Job drawing, mm, ordinate dimensions from the low corner. One solid piece. Give positions to 0.01 mm unless a question says otherwise; leave off trailing zeros. Order: outer loops, then holes, each group sorted by start corner. A loop starts at its lowest first (then second) coordinate and runs counter-clockwise, first axis right, second up. Notation, with made-up numbers: (76, 4.5) -> (116, 4.5) arc R31 cw to (116, 36.5) -> close; hole circle Ø11 at (49.25, 81). An arc over 180 degrees is marked (long way). Write item = value, one per line. Start each with the question number.
(1) Saw through at D-D, the plane z = 55.1. List the corners of the cut face in (x, y), then the cut area to 3 significant figures.
(2) Saw through at B-B, the plane z = 6.9. List the corners of the cut face in (x, y).
(3) Flat gauge pins, fed straight in: pin 1 (4 mm diameter, centred on x = 67, z = 27.5, fed in from +Y); pin 2 (0.9 mm diameter, centred on x = 6, z = 7, fed in from +Y); pin 3 (0.8 mm diameter, centred on x = 8, y = 3.5, fed in from +Z). Where does each tip first touch, or does it go through?
(4) Saw through at C-C, the plane x = 9. List the corners of the cut face in (y, z), then the cut area to 3 significant figures.
(5) Probe line 1 along X through (y, z) = (3.95, 6.9); line 2 along Z through (x, y) = (65.6, 3.95); line 3 along X through (y, z) = (4.75, 43). List the from-to ranges inside material, lowest first. Write a range as from..to.
(6) Saw through at A-A, the plane y = 3. List the corners of the cut face in (x, z).
(7) Two-plate mould, pull along X, no slides. Class the marked faces 1, 2, 3 and 4: pulls with the +X half, pulls with the -X half, needs draft (parallel to the pull), parting line crosses it, or undercut.
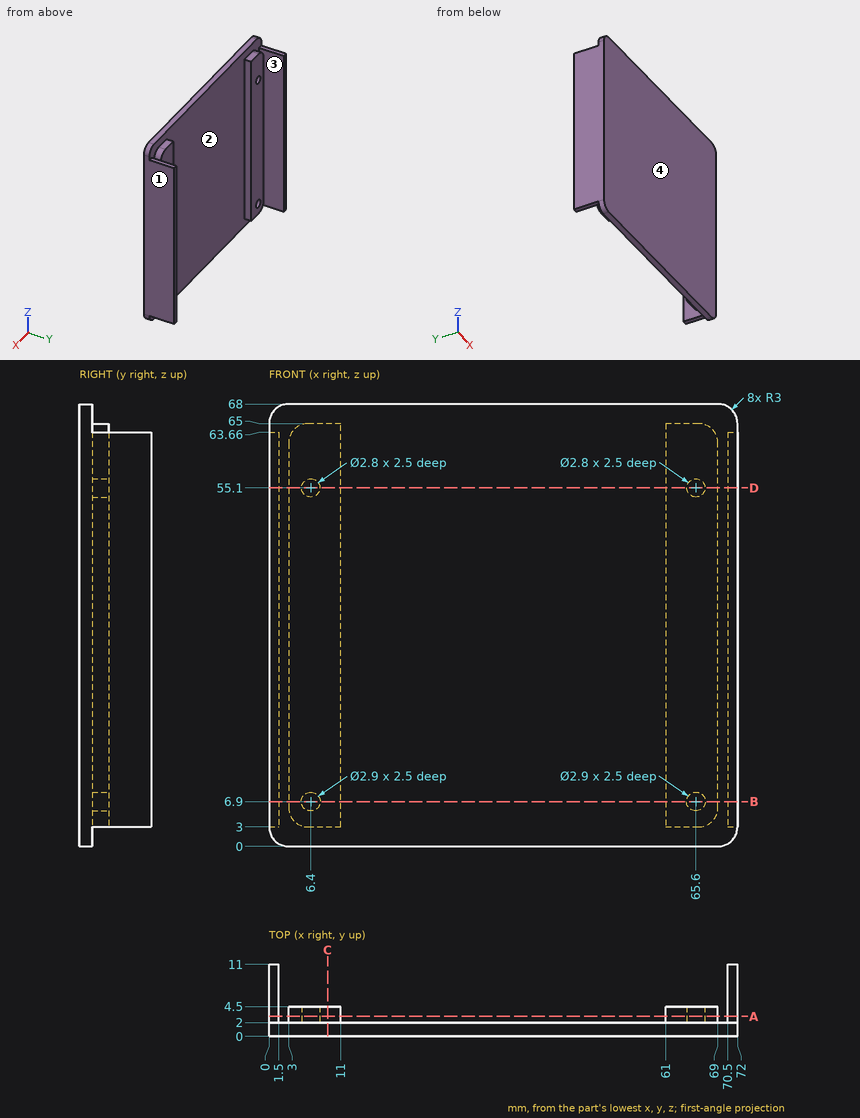
Results list:
q1.outline = (0, 0) -> (72, 0) -> (72, 11) -> (70.5, 11) -> (70.5, 2) -> (69, 2) -> (69, 4.5) -> (67, 4.5) -> (67, 2) -> (64.2, 2) -> (64.2, 4.5) -> (61, 4.5) -> (61, 2) -> (11, 2) -> (11, 4.5) -> (7.8, 4.5) -> (7.8, 2) -> (5, 2) -> (5, 4.5) -> (3, 4.5) -> (3, 2) -> (1.5, 2) -> (1.5, 11) -> (0, 11) -> close
q1.area = 197 mm^2
q2.outline = (0, 0) -> (72, 0) -> (72, 11) -> (70.5, 11) -> (70.5, 2) -> (69, 2) -> (69, 4.5) -> (67.05, 4.5) -> (67.05, 2) -> (64.15, 2) -> (64.15, 4.5) -> (61, 4.5) -> (61, 2) -> (11, 2) -> (11, 4.5) -> (7.85, 4.5) -> (7.85, 2) -> (4.95, 2) -> (4.95, 4.5) -> (3, 4.5) -> (3, 2) -> (1.5, 2) -> (1.5, 11) -> (0, 11) -> close
q3.pin_1 = 4.5
q3.pin_2 = 2
q3.pin_3 = 65
q4.outline = (0, 0) -> (2, 0) -> (2, 3) -> (4.5, 3) -> (4.5, 65) -> (2, 65) -> (2, 68) -> (0, 68) -> close
q4.area = 291 mm^2
q5.line_1 = 0..1.5, 3..4.95, 7.85..11, 61..64.15, 67.05..69, 70.5..72
q5.line_2 = 3..5.45, 8.35..53.7, 56.5..65
q5.line_3 = 0..1.5, 70.5..72
q6.outline = (0, 3) -> (1.5, 3) -> (1.5, 63.66) -> (0, 63.66) -> close; (3, 6) arc R3 ccw to (6, 3) -> (11, 3) -> (11, 65) -> (6, 65) arc R3 ccw to (3, 62) -> close; (61, 3) -> (66, 3) arc R3 ccw to (69, 6) -> (69, 62) arc R3 ccw to (66, 65) -> (61, 65) -> close; (70.5, 3) -> (72, 3) -> (72, 63.66) -> (70.5, 63.66) -> close; hole circle Ø2.9 at (6.4, 6.9); hole circle Ø2.8 at (6.4, 55.1); hole circle Ø2.9 at (65.6, 6.9); hole circle Ø2.8 at (65.6, 55.1)
q7.face_1 = pulls with the +X half
q7.face_2 = undercut
q7.face_3 = undercut
q7.face_4 = needs draft
